Input: part model. Units: mm. Frame: model coordinates. A direction names the side the tool comes from. Give positions to 0.01 mm unless a question says otherwise; leave off trailing zeros. Loops run counter-clockwise (first coordinate to the right, second up) from the corner with the lowest first, then second, coordinate; pieces in that order, holes last. Notation, with made-up numbers: (-38.75, 21.25) - (-17.75, 21.25) arc R13 cw to (-17.75, 43.25) - close; hole circle Ø10 at (37, 42.5). An arc over 180 degrees is marked (long way). Answer as a JSON object with one key per item and string values.
from build123d import *

# Parameters (mm, degrees)
SKETCH1_W                = 13.5
SKETCH1_H                = 27
MAIN_DEPTH               = 3.675
SKETCH2_R                = 2.75
BACKCABLEHOLE_DEPTH      = 8.5
SKETCH3_W                = 5.7
SKETCH3_H                = 5.7
FRONTCONNECTORHOLE_DEPTH = 8.5
MAINHOOK_DEPTH           = 1.75
SKETCH5_W                = 1.1
SKETCH5_H                = 1.1
BOTTOMLINE_DEPTH         = 4.5
SKETCH6_W                = 3.3
SKETCH6_H                = 1.1
SIDEHOOK_DEPTH           = 1.1


with BuildPart() as part:
    # Sketch1 → Main (new body, symmetric)
    with BuildSketch(Plane.XY):
        Rectangle(SKETCH1_W, SKETCH1_H)
    extrude(amount=MAIN_DEPTH, both=True)

    # Sketch2 → BackCableHole (cut)
    with BuildSketch(Plane(origin=(0, -13.5, 0), x_dir=(-1, 0, 0), z_dir=(0, -1, 0))):
        with Locations((3, 0)):
            Circle(SKETCH2_R)
        with Locations((-3, 0)):
            Circle(SKETCH2_R)
    extrude(amount=-BACKCABLEHOLE_DEPTH, mode=Mode.SUBTRACT)

    # Sketch3 → FrontConnectorHole (cut)
    with BuildSketch(Plane(origin=(0, 13.5, 0), x_dir=(1, 0, 0), z_dir=(0, 1, 0))):
        with Locations((-3.2, 0)):
            Rectangle(SKETCH3_W, SKETCH3_H)
        with BuildLine():
            Line((6.05, -2.85), (0.35, -2.85))
            Line((0.35, -2.85), (0.35, 0))
            ThreePointArc((0.35, 0), (3.2, 2.85), (6.05, 0))
            Line((6.05, 0), (6.05, -2.85))
        make_face()
    extrude(amount=-FRONTCONNECTORHOLE_DEPTH, mode=Mode.SUBTRACT)

    # Sketch4 → MainHook (add, symmetric)
    with BuildSketch(Plane(origin=(0, 0, 0), x_dir=(0, 0, -1), z_dir=(1, 0, 0))):
        Polygon((-3.675, 13.5), (-5.175, 11), (-3.675, 11), align=None)
    extrude(amount=MAINHOOK_DEPTH, both=True)

    # Sketch5 → BottomLine (add, symmetric)
    with BuildSketch(Plane(origin=(0, 0, 0), x_dir=(0, 0, -1), z_dir=(1, 0, 0))):
        with Locations((4.225, 0.35)):
            Rectangle(SKETCH5_W, SKETCH5_H)
    extrude(amount=BOTTOMLINE_DEPTH, both=True)

    # Sketch6 → SideHook (add)
    with BuildSketch(Plane.XY.offset(3.675)):
        with Locations((-5.1, 0.05)):
            Rectangle(SKETCH6_W, SKETCH6_H)
        with Locations((5.1, 0.05)):
            Rectangle(SKETCH6_W, SKETCH6_H)
    extrude(amount=SIDEHOOK_DEPTH)


solid = part.part
Item 1: Cut plane D-D (y = 4.5). Return loops of the section in (x, z) (3 decimals).
Geometry check:
{"outline": "(-6.75, -3.675) - (6.75, -3.675) - (6.75, 3.675) - (-6.75, 3.675) - close"}
Item 2: Cut plane C-C (z = -2). Return loops of the section in (x, y).
Geometry check:
{"outline": "(-6.75, -13.5) - (-4.89, -13.5) - (-4.89, -5) - (-1.11, -5) - (-1.11, -13.5) - (1.11, -13.5) - (1.11, -5) - (4.89, -5) - (4.89, -13.5) - (6.75, -13.5) - (6.75, 13.5) - (5.23, 13.5) - (5.23, 5) - (1.17, 5) - (1.17, 13.5) - (-0.35, 13.5) - (-0.35, 5) - (-6.05, 5) - (-6.05, 13.5) - (-6.75, 13.5) - close"}
Item 3: Material intervals for line 1 (X direction, y = -8, z = 0); line 2 (Z direction, x = -3, y = -11) (3 decimals); line 3 (Z direction, x = -3.75, y = 9.25) (3 decimals), sorted ascending. Write a range as [from, to].
Geometry check:
{"line 1": "x = [-6.75, -5.75], [-0.25, 0.25], [5.75, 6.75]", "line 2": "z = [-3.675, -2.75], [2.75, 3.675]", "line 3": "z = [-3.675, -2.85], [2.85, 3.675]"}
Item 4: Cut plane A-A (y = 7.75). Return loops of the section in (x, z) (3 decimals).
Geometry check:
{"outline": "(-6.75, -3.675) - (6.75, -3.675) - (6.75, 3.675) - (-6.75, 3.675) - close; hole (-6.05, -2.85) - (-0.35, -2.85) - (-0.35, 2.85) - (-6.05, 2.85) - close; hole (0.35, 0) arc R2.85 ccw to (6.05, 0) - (6.05, 2.85) - (0.35, 2.85) - close"}
Item 5: Access query for faces 5 (the face through (0, 0.9, -4)), 6 (the face through (3, -5, 0)), 7 (the face through (-4.5, 0, -4)), 8 (the face through (0.35, 9, 1)), 9 (the face through (3.45, 0, 4)). Directions: +Z, -Z, +X, -X, +Y, -Y. A direction counts if a zero-diameter tool reaches every point of the face in a straight line with its end or side. Return the directions, or none.
Geometry check:
{"face 5": "-Z, +X, -X, +Y", "face 6": "-Y", "face 7": "-Z, -X, +Y, -Y", "face 8": "+Y", "face 9": "+Z, +Y, -Y"}
Item 6: Mould query, pull axis X, two halves, no side actions, for faces 1 (the face through (4.5, 0, -4)), 2 (the face through (-3, 5, 0)), 3 (the face through (5, 0.6, 4)), 4 (the face through (6.05, 9, 1)). Classes: released by +X, released by -X, zero draft, split by the parting line, or undercut.
Geometry check:
{"face 1": "released by +X", "face 2": "undercut", "face 3": "zero draft", "face 4": "undercut"}
Item 7: Contact query for flat-ended pins moving along their axis: P1, Ø4.5, axis at x = -4.5, z = 0, coming from the +Y side; P2, Ø1.5, axis at x = 4, y = 4, coming from the -Z side (3 decimals); P3, Ø8, axis at x = -2, y = -4.5, coming from the +Z side (3 decimals); P4, Ø3, axis at x = 3.5, z = 0, coming from the +Y side. Output: stop coordinate, or through.
Geometry check:
{"P1": "stops at y = 13.5", "P2": "stops at z = -3.675", "P3": "stops at z = 3.675", "P4": "stops at y = 5"}
Item 8: Cut plane B-B (x = -3). Return loops of the section in (y, z) (3 decimals), then the cut area to 3 significant figures.
Geometry check:
{"outline": "(-13.5, -3.675) - (-0.2, -3.675) - (-0.2, -4.775) - (0.9, -4.775) - (0.9, -3.675) - (13.5, -3.675) - (13.5, -2.85) - (5, -2.85) - (5, 2.85) - (13.5, 2.85) - (13.5, 3.675) - (-13.5, 3.675) - (-13.5, 2.75) - (-5, 2.75) - (-5, -2.75) - (-13.5, -2.75) - close", "area": "104 mm2"}
